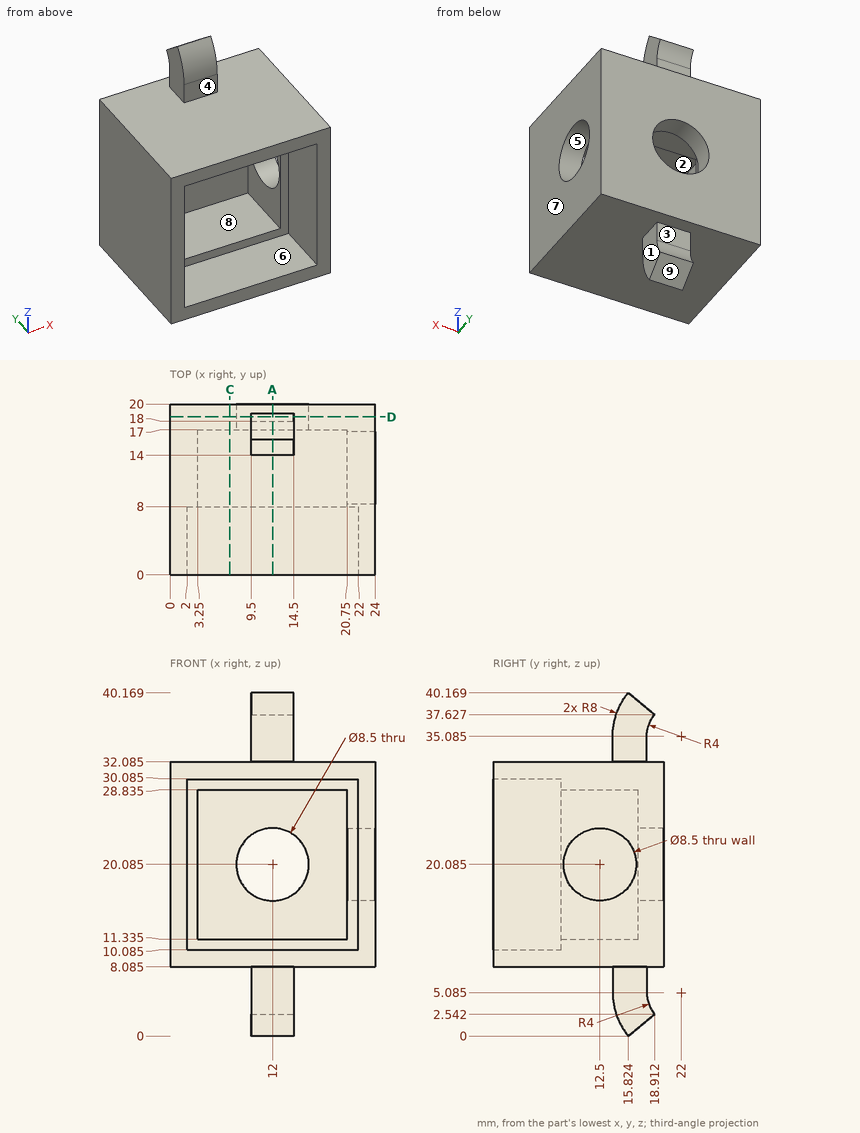
For this review, use the dimensioned drawing (mm, ordinates from the lowest corner) and the shaded views. A direction names the side the tool comes from. Round coordinates to 2 decimals unless told otherwise and drop trailing zeros. Write each loop counter-clockwise with the first axis right and the second up, starting at its lowest first coordinate (ties: lowest second). Pieces come first, ordered by that corner, then holes. Notation, with made-up numbers: (-22, 87) -> (-14, 87) arc R20 ccw to (-14, 106) -> close; hole circle Ø9 at (72.25, 79). An arc over 180 degrees is marked (long way). One line per item, written item: value. Start each with the question number.
Q1. To check wall thickness, follow probe 1 along X at (y, z) = (2.25, 30); probe 2 along X at (y, z) = (16, 23); probe 3 along Z at (x, y) = (13, 10) (1 decimal). State the ranges of each line that lie inside material, in increasing order.
Q2. Add section C-C (x = 7). Give the boundary of the cut face in (y, z) (1 decimal).
Q3. Insertion check: P1, Ø6, axis at x = 20.5, y = 13, coming from the +Z side (1 decimal); P2, Ø1.5, axis at y = 17, z = 2.5, coming from the -X side; P3, Ø4.5, axis at y = 11.5, z = 20.5, coming from the +X side; P4, Ø7.5, axis at x = 12, z = 20.08, coming from the -Y side. Each pin has a flat end and moves straight along its axis. Give the tip position at first contact, or say it passes through.
Q4. Tool access review of the marked faces 1, 2, 3, 4 and 5: name each direction out of +Z, -Z, +X, -X, +Y, -Y from which nothing blocks a thin tool from reaching the whole face with its end or side.
Q5. Add section D-D (y = 18.5). State how many separate pieces and enclosed holes the cut face has, then the cut area to 3 significant figures.
Q6. The part is to be moulded in two halves that separate along Z. For the marked faces 6, 7, 8 and 9, say which applies: pulls with the +Z half, pulls with the -Z half, needs draft (parallel to the pull), parting line crosses it, or undercut.
Q7. Add section A-A (x = 12). Give the boundary of the cut face in (y, z) (1 decimal), then the cut area to 3 significant figures.
Response:
1. probe 1: x = 0 to 2, 22 to 24
1. probe 2: x = 0 to 3.25, 20.75 to 24
1. probe 3: z = 8.1 to 11.3, 28.8 to 32.1
2. outline: (0, 8.1) -> (20, 8.1) -> (20, 32.1) -> (0, 32.1) -> (0, 30.1) -> (8, 30.1) -> (8, 28.8) -> (17, 28.8) -> (17, 11.3) -> (8, 11.3) -> (8, 10.1) -> (0, 10.1) -> close
3. P1: stops at z = 32.1
3. P2: stops at x = 9.5
3. P3: stops at x = 3.25
3. P4: passes through
4. face 1: -Z, +X, +Y, -Y
4. face 2: -Y
4. face 3: +X, -X, +Y
4. face 4: +Z, +X, -X, -Y
4. face 5: +X
5. separate pieces: 3
5. enclosed holes: 1
5. area: 529 mm^2
6. face 6: undercut
6. face 7: needs draft
6. face 8: undercut
6. face 9: pulls with the -Z half
7. outline: (0, 8.1) -> (14, 8.1) -> (14, 5.1) arc R8 ccw to (15.8, 0) -> (18.9, 2.5) arc R4 cw to (18, 5.1) -> (18, 8.1) -> (20, 8.1) -> (20, 15.8) -> (17, 15.8) -> (17, 11.3) -> (8, 11.3) -> (8, 10.1) -> (0, 10.1) -> close; (0, 30.1) -> (8, 30.1) -> (8, 28.8) -> (17, 28.8) -> (17, 24.3) -> (20, 24.3) -> (20, 32.1) -> (18, 32.1) -> (18, 35.1) arc R4 cw to (18.9, 37.6) -> (15.8, 40.2) arc R8 ccw to (14, 35.1) -> (14, 32.1) -> (0, 32.1) -> close
7. area: 194 mm^2
